Design review of the part built by this model. Coordinates are the model's own, in mm. Face numbers are marked on the shaded views. A direction names the side the tool comes from. Round coordinates to 2 decimals unless told otherwise and drop trailing zeros. Loops run counter-clockwise (first coordinate to the right, second up) from the corner with the lowest first, then second, coordinate; pieces in that order, holes last. Notation, with made-up numbers: M -21.5,76.5 L 11.5,76.5 A13 ccw 11.5,96.5 Z; hole C -24,14 d7. An arc over 180 degrees is marked long. Use a Markdown table: item, result.
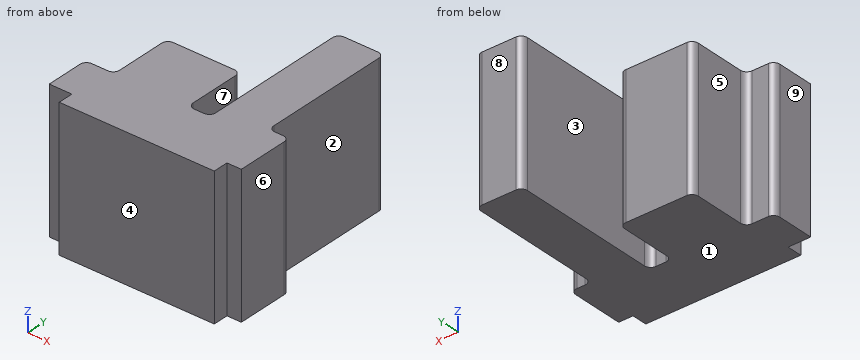
from build123d import *

# Parameters (mm, degrees)
Y_KSEKLIK_EKSTR_ZYON2_DEPTH = 66


with BuildPart() as part:
    # Çizim5 → Yükseklik-Ekstrüzyon2 (new body)
    with BuildSketch(Plane.XY):
        with BuildLine():
            Line((3, 27.837901934), (10.723277294, 27.837901934))
            ThreePointArc((10.723277294, 27.837901934), (12.844597638, 28.716581591), (13.723277294, 30.837901934))
            Line((13.723277294, 30.837901934), (13.723277294, 54.860494767))
            ThreePointArc((13.723277294, 54.860494767), (14.60195695, 56.98181511), (16.723277294, 57.860494767))
            Line((16.723277294, 57.860494767), (45.588223809, 57.860494767))
            ThreePointArc((45.588223809, 57.860494767), (47.709544152, 56.98181511), (48.588223809, 54.860494767))
            Line((48.588223809, 54.860494767), (48.588223809, 30.837901934))
            ThreePointArc((48.588223809, 30.837901934), (49.466903465, 28.716581591), (51.588223809, 27.837901934))
            Line((51.588223809, 27.837901934), (56.24140191, 27.837901934))
            ThreePointArc((56.24140191, 27.837901934), (58.362722254, 28.716581591), (59.24140191, 30.837901934))
            Line((59.24140191, 30.837901934), (59.24140191, 97.571673858))
            ThreePointArc((59.24140191, 97.571673858), (60.120081567, 99.692994202), (62.24140191, 100.571673858))
            Line((62.24140191, 100.571673858), (78.193405271, 100.571673858))
            ThreePointArc((78.193405271, 100.571673858), (80.314725615, 99.692994202), (81.193405271, 97.571673858))
            Line((81.193405271, 97.571673858), (81.193405271, 37.61719709))
            ThreePointArc((81.193405271, 37.61719709), (82.072084928, 35.495876747), (84.193405271, 34.61719709))
            Line((84.193405271, 34.61719709), (88.033262194, 34.61719709))
            ThreePointArc((88.033262194, 34.61719709), (90.154582538, 33.738517434), (91.033262194, 31.61719709))
            Line((91.033262194, 31.61719709), (91.033262194, 7.220315017))
            Line((91.033262194, 7.220315017), (84.193405271, 7.220315017))
            Line((84.193405271, 7.220315017), (84.193405271, 0))
            Line((84.193405271, 0), (10.723277294, 0))
            Line((10.723277294, 0), (10.723277294, 7.220315017))
            Line((10.723277294, 7.220315017), (0, 7.220315017))
            Line((0, 7.220315017), (0, 24.837901934))
            ThreePointArc((0, 24.837901934), (0.878679656, 26.959222278), (3, 27.837901934))
        make_face()
    extrude(amount=Y_KSEKLIK_EKSTR_ZYON2_DEPTH)


solid = part.part
1. Take a section at C-C on x = 9. Give the boundary of the cut face in (y, z).
Check values:
| item | result |
|---|---|
| outline | M 7.22,0 L 27.84,0 L 27.84,66 L 7.22,66 Z |
2. Take a section at D-D on y = 70.5. Give the boundary of the cut face in (x, z), and give its area (3 significant figures).
Check values:
| item | result |
|---|---|
| outline | M 59.24,0 L 81.19,0 L 81.19,66 L 59.24,66 Z |
| area | 1,450 mm² |
3. Take a section at B-B on z = 22. Give the boundary of the cut face in (x, y).
Check values:
| item | result |
|---|---|
| outline | M 0,7.22 L 10.72,7.22 L 10.72,0 L 84.19,0 L 84.19,7.22 L 91.03,7.22 L 91.03,31.62 A3 ccw 88.03,34.62 L 84.19,34.62 A3 cw 81.19,37.62 L 81.19,97.57 A3 ccw 78.19,100.57 L 62.24,100.57 A3 ccw 59.24,97.57 L 59.24,30.84 A3 cw 56.24,27.84 L 51.59,27.84 A3 cw 48.59,30.84 L 48.59,54.86 A3 ccw 45.59,57.86 L 16.72,57.86 A3 ccw 13.72,54.86 L 13.72,30.84 A3 cw 10.72,27.84 L 3,27.84 A3 ccw 0,24.84 Z |
4. Wall thickness on line 1 along X through (y, z) = (50.5, 36); line 2 along X through (y, z) = (32, 62); line 3 along X through (y, z) = (72, 53): over which ranges is each line inside the solid? List them lowest first. Write a range as from..to.
Check values:
| item | result |
|---|---|
| line 1 | x = 13.72..48.59, 59.24..81.19 |
| line 2 | x = 13.72..48.59, 59.24..91.01 |
| line 3 | x = 59.24..81.19 |
5. Machinability: for the marked faces 1, 2, 3, 4 and 5, which of the approach directions +Z, -Z, +X, -X, +Y, -Y give a long, thin tool a straight path to every point of the face, cutting with its end or side? Answer none if there is none.
Check values:
| item | result |
|---|---|
| face 1 | -Z, +X, -X, +Y, -Y |
| face 2 | +Z, -Z, +X, +Y |
| face 3 | +Z, -Z, +Y |
| face 4 | +Z, -Z, +X, -X, -Y |
| face 5 | +Z, -Z, -X, +Y |
6. Insertion check: pin 1 (20 mm diameter, centred on y = 59, z = 17.5, fed in from -X); pin 2 (6 mm diameter, centred on y = 2.5, z = 35.5, fed in from +X); pin 3 (8.5 mm diameter, centred on x = 7, z = 37, fed in from +Y). Each pin has a flat end and moves straight along its axis. Give the tip position at first contact, or say it passes through.
Check values:
| item | result |
|---|---|
| pin 1 | stops at x = 13.72 |
| pin 2 | stops at x = 84.19 |
| pin 3 | stops at y = 27.88 |
7. Take a section at A-A on y = 39. Give the boundary of the cut face in (x, z).
Check values:
| item | result |
|---|---|
| outline | M 13.72,0 L 48.59,0 L 48.59,66 L 13.72,66 Z; M 59.24,0 L 81.19,0 L 81.19,66 L 59.24,66 Z |
8. The part is to be moulded in two halves that separate along X. For the marked faces 6, 7, 8 and 9, say which applies: pulls with the +X half, pulls with the -X half, needs draft (parallel to the pull), parting line crosses it, or undercut.
Check values:
| item | result |
|---|---|
| face 6 | pulls with the +X half |
| face 7 | undercut |
| face 8 | needs draft |
| face 9 | pulls with the -X half |
